Autodesk Inventor part; units mm, degrees
ref_plane "YZ Plane" through (0, 0, 0) normal (1, 0, 0) x (0, 1, 0)
ref_plane "XZ Plane" through (0, 0, 0) normal (0, 1, 0) x (-1, 0, 0)
ref_plane "XY Plane" through (0, 0, 0) normal (0, 0, 1) x (1, 0, 0)
sketch "Esboço1" plane through (0, 0, 0) normal (0, 0, 1) x (1, 0, 0)
  line L0 (0, 0) -> (32, 0)
  line L1 (32, 0) -> (32, 26)
  line L2 (32, 26) -> (0, 26)
  line L3 (0, 26) -> (0, 0)
  dimension "d0" = 32
  dimension "d1" = 26
extrude "Extrusão1" add sketch "Esboço1" against normal blind 16
shell "Casca1" thickness 2.5 removed faces 1 at (21.3333, 26, -10.6667)
sketch "Esboço2" plane through (0, 0, -16) normal (0, 0, -1) x (-1, 0, 0)
  line L0 (0, 0) -> (0, 26)
  line L1 (0, 21) -> (12, 21)
  line L2 (12, 21) -> (12, 5)
  line L3 (12, 5) -> (0, 5)
  line L4 (0, 5) -> (0, 21)
  line L5 (-32, 0) -> (0, 0)
  line L6 (-32, 26) -> (-32, 0)
  line L7 (-32, 21) -> (-44, 21)
  line L8 (-44, 21) -> (-44, 5)
  line L9 (-44, 5) -> (-32, 5)
  line L10 (-32, 5) -> (-32, 21)
  point P0 (-32, 5)
  point P1 (0, 5)
  dimension "d5" = 12
  dimension "d6" = 16
  dimension "d7" = 5
  dimension "d8" = 12
  dimension "d18" = 16
  dimension "d19" = 5
extrude "Extrusão2" add sketch "Esboço2" against normal blind 3
sketch "Esboço3" plane through (0, 0, -16) normal (0, 0, -1) x (-1, 0, 0)
  circle A0 centre (5.5, 13) radius 2.5
  line L0 (12, 5) -> (12, 21)
  circle A1 centre (-37.5, 13) radius 2.5
  line L1 (-44, 21) -> (-44, 5)
  point P0 (0, 0)
  dimension "d11" = 5
  dimension "d12" = 6.5
  dimension "d13" = 5
  dimension "d14" = 6.5
extrude "Extrusão3" cut sketch "Esboço3" against normal blind 3
fillet "Arredondamento1" radius 7 4 edges at (44, 21, -14.5) (44, 5, -14.5) (-12, 5, -14.5) (-12, 21, -14.5)
fillet "Arredondamento2" radius 1 2 edges at (32, 13, 0) (0, 13, 0)
sketch "Esboço4" plane through (32, 5, -13) normal (1, 0, 0) x (0, 0, -1)
  circle A0 centre (-6, 1.428) radius 1.25
  line L0 (0, 0) -> (0, 7)
  point P0 (-13, -5)
  dimension "d21" = 2.5
  dimension "d22" = 6
extrude "Extrusão4" cut sketch "Esboço4" against normal blind 36.75
properties part number "caixa do fusivel"
Verification items for the finished model (mm, model axes). A direction names the side the tool comes from. Give positions to 0.01 mm unless a question says otherwise; leave off trailing zeros. Order: outer loops, then holes, each group sorted by start corner. A loop starts at its lowest first (then second) coordinate and runs counter-clockwise, first axis right, second up. Notation, with made-up numbers: M -33,30 L -17,30 A6 cw -17,35 Z; hole C 30.25,49.5 d1. An arc over 180 degrees is marked long. Answer as a JSON object with one key per item and string values. Group by question number.
1) Access from +Z, -Z, +X, -X, +Y, -Y to the whole of each face (thin tool, end or side, straight path). Record for faces 4 (the face through (16, 14, -2.5)), 5 (the face through (-3, 11, -13)), 6 (the face through (39.4, 14.9, -13)).
2) Cross-section at A-A (y = 13). Enter the section's corners in (x, z).
3) Mould release check, pull along Y, two halves, no side actions. Record for faces 1 (the face through (16, 13, -16)), 2 (the face through (41.9, 7, -14.5)), 3 (the face through (1.267, 5.208, -6.729)): released by +Y, released by -Y, zero draft, split by the parting line, or undercut.
4) Depth check by flat-ended pin: pin 1 Ø0.9 at (x, z) = (34.5, -15) entering from +Y; pin 2 Ø8 at (x, y) = (-5.5, 13) entering from -Z; pin 3 Ø1 at (x, y) = (34, 3.5) entering from -Z; pin 4 Ø9 at (y, z) = (10.5, -7.5) entering from -X. Enter the tip coordinate at first touch or a pass-through.
5) Cross-section at B-B (y = 22.5). Enter the section's corners in (x, z), then the cut area to 3 significant figures.
6) Cross-section at C-C (x = 24.5). Enter the section's corners in (y, z), then the cut area to 4 significant figures.
7) Cross-section at D-D (y = 17). Enter the section's corners in (x, z).
8) Scan lines: line 1 along X through (y, z) = (22.75, -3.5); line 2 along Z through (x, y) = (20.5, 24.5); line 3 along Y through (x, z) = (30.2, -7). Record each from-to range of solid material in increasing order. Write a range as [from, to].
Result sheet:
{
 "1": {"face 4": "+Y", "face 5": "+Z, -X, +Y, -Y", "face 6": "+Z, +X, +Y, -Y"},
 "2": {"outline": "M -12,-16 L -8,-16 L -8,-13 L -12,-13 Z; M -3,-16 L 35,-16 L 35,-13 L 32,-13 L 32,-1 A1 ccw 31,0 L 1,0 A1 ccw 0,-1 L 0,-13 L -3,-13 Z; M 40,-16 L 44,-16 L 44,-13 L 40,-13 Z; hole M 2.5,-13.5 L 29.5,-13.5 L 29.5,-2.5 L 2.5,-2.5 Z"},
 "3": {"face 1": "zero draft", "face 2": "released by -Y", "face 3": "undercut"},
 "4": {"pin 1": "stops at y = 21", "pin 2": "stops at z = -16", "pin 3": "passes through", "pin 4": "stops at x = 0"},
 "5": {"outline": "M 0,-16 L 32,-16 L 32,-1 A1 ccw 31,0 L 1,0 A1 ccw 0,-1 Z; hole M 2.5,-13.5 L 29.5,-13.5 L 29.5,-2.5 L 2.5,-2.5 Z", "area": "215 mm2"},
 "6": {"outline": "M 0,-16 L 26,-16 L 26,-13.5 L 2.5,-13.5 L 2.5,-2.5 L 26,-2.5 L 26,0 L 0,0 Z", "area": "157.5 mm2"},
 "7": {"outline": "M -11.32,-16 L 43.32,-16 L 43.32,-13 L 32,-13 L 32,-1 A1 ccw 31,0 L 1,0 A1 ccw 0,-1 L 0,-13 L -11.32,-13 Z; hole M 2.5,-13.5 L 29.5,-13.5 L 29.5,-2.5 L 2.5,-2.5 Z"},
 "8": {"line 1": "x = [0, 2.5], [29.5, 32]", "line 2": "z = [-16, -13.5], [-2.5, 0]", "line 3": "y = [0, 5.18], [7.68, 26]"}
}
